Verification items for the finished model (mm, model axes). A direction names the side the tool comes from. Give positions to 0.01 mm unless a question says otherwise; leave off trailing zeros. Write each loop counter-clockwise with the first axis right and the second up, starting at its lowest first coordinate (ties: lowest second). Pieces come first, ordered by that corner, then holes. Notation, with made-up numbers: M 66.25,-14 L 77.25,-14 A17 ccw 77.25,-4 Z; hole C 89.5,40.5 d1. An arc over 180 degrees is marked long. Answer as a JSON object with one key per item and string values.
```python
from build123d import *

# Parameters (mm, degrees)
F0_W      = 76.2
F0_H      = 76.2
F1_DEPTH  = 19.05
F2_R      = 25.4
F3_DEPTH  = 76.2
F4_W      = 76.2
F4_H      = 76.2
F4_R      = 25.4
F5_DEPTH  = 19.05
F6_R      = 25.4
F7_DEPTH  = 19.05
F9_R      = 19.05
F10_DEPTH = 114.3
F8_R      = 19.05
F11_DEPTH = 608.076
F13_R     = 6.35
F14_DEPTH = 50.546


with BuildPart() as f1:
    # F0 (on Right) → F1 (new body)
    with BuildSketch(Plane.YZ):
        Rectangle(F0_W, F0_H)
    extrude(amount=F1_DEPTH)

    # F2 (on face) → F3 (join)
    with BuildSketch(Plane(origin=(0, 0, 0), x_dir=(0, -1, 0), z_dir=(-1, 0, 0))):
        Circle(F2_R)
    extrude(amount=F3_DEPTH)


with BuildPart() as f5:
    # F4 (on face) → F5 (new body)
    with BuildSketch(Plane(origin=(-76.2, 0, 0), x_dir=(0, -1, 0), z_dir=(-1, 0, 0))):
        Rectangle(F4_W, F4_H)
        Circle(F4_R, mode=Mode.SUBTRACT)
    extrude(amount=F5_DEPTH)


with BuildPart() as f7:
    # F6 (on face) → F7 (new body)
    with BuildSketch(Plane(origin=(-76.2, 0, 0), x_dir=(0, -1, 0), z_dir=(-1, 0, 0))):
        Circle(F6_R)
    extrude(amount=F7_DEPTH)


with BuildPart() as f10_tool:
    # F9 (on face) → F10 (new body)
    with BuildSketch(Plane.YZ.offset(19.05)):
        Circle(F9_R)
    extrude(amount=-F10_DEPTH)


with BuildPart() as f1_1:
    add(f1.part)

    # F10: cut by f10_tool
    add(f10_tool.part, mode=Mode.SUBTRACT)

    # F8 (on face) → F11 (cut)
    with BuildSketch(Plane(origin=(-95.25, 0, 0), x_dir=(0, -1, 0), z_dir=(-1, 0, 0))):
        Circle(F8_R)
    extrude(amount=-F11_DEPTH, mode=Mode.SUBTRACT)


with BuildPart() as f7_1:
    add(f7.part)

    # F10: cut by f10_tool
    add(f10_tool.part, mode=Mode.SUBTRACT)


with BuildPart() as f5_1:
    add(f5.part)

    # F12: union F7, F1
    add(f7_1.part)
    add(f1_1.part)

    # F13 (on face) → F14 (cut)
    with BuildSketch(Plane(origin=(-95.25, 0, 0), x_dir=(0, -1, 0), z_dir=(-1, 0, 0))):
        with Locations((-29.2046008315, -27.7056374614)):
            Circle(F13_R)
        with Locations((27.7061383014, 29.4438616986)):
            Circle(F13_R)
        with BuildLine():
            ThreePointArc((-23.0938616986, 29.4438616986), (-27.0138219031, 35.3104967301), (-33.9339897591, 33.9339897591))
            Line((-33.9339897591, 33.9339897591), (-24.9537336381, 24.9537336381))
            ThreePointArc((-24.9537336381, 24.9537336381), (-23.5772266672, 27.0138219031), (-23.0938616986, 29.4438616986))
        make_face()
        with BuildLine():
            ThreePointArc((23.3369908748, -23.3369908748), (23.455271108, -32.1957655219), (32.3140457551, -32.3140457551))
            Line((32.3140457551, -32.3140457551), (23.3369908748, -23.3369908748))
        make_face()
        with BuildLine():
            Line((23.3369908748, -23.3369908748), (32.3140457551, -32.3140457551))
            ThreePointArc((32.3140457551, -32.3140457551), (33.7790689323, -30.213783607), (34.2953991685, -27.7056374614))
            ThreePointArc((34.2953991685, -27.7056374614), (30.2968994699, -21.8070828645), (23.3369908748, -23.3369908748))
        make_face()
    extrude(amount=-F14_DEPTH, mode=Mode.SUBTRACT)


solid = f5_1.part
```
1) Section check D-D on x = 8.5. Record the boundary of the cut face in (y, z).
Completed:
{"outline": "M -38.1,-38.1 L 38.1,-38.1 L 38.1,38.1 L -38.1,38.1 Z; hole C 0,0 d38.1"}
2) Thickness scan on L1, parallel to X at y = 28.5, z = -13; L2, parallel to Z at x = -86, y = -22.5; L3, parallel to Z at x = -24.5, y = 0. Record the ranges inside material, lowest first.
Completed:
{"L1": "x = -95.25 to -76.2, 0 to 19.05", "L2": "z = -38.1 to -30.97, -24.44 to 25.81, 33.08 to 38.1", "L3": "z = -25.4 to -19.05, 19.05 to 25.4"}
3) Go/stop test with flat-tipped pins: pin 1 (6 mm diameter, centred on x = -22, y = -15.5, fed in from -Z); pin 2 (1 mm diameter, centred on x = -28, z = 18, fed in from +Y); pin 3 (7.5 mm diameter, centred on y = 29.2, z = -27.71, fed in from -X). Record where each tip stops, or that it passes through.
Completed:
{"pin 1": "stops at z = -22.11", "pin 2": "stops at y = 18.41", "pin 3": "stops at x = 0"}
4) Section check B-B on x = -85. Record the boundary of the cut face in (y, z).
Completed:
{"outline": "M -38.1,-38.1 L 38.1,-38.1 L 38.1,38.1 L -38.1,38.1 Z; hole C -27.95,-27.71 d12.7; hole C -27.71,29.44 d12.7; hole C 0,0 d38.1; hole C 29.2,-27.71 d12.7; hole M 24.95,24.95 L 33.93,33.93 A6.35 ccw Z"}
5) Section check A-A on y = 0. Record the boundary of the cut face in (x, z), and give its area (3 significant figures).
Completed:
{"outline": "M -95.25,-38.1 L -76.2,-38.1 L -76.2,-25.4 L 0,-25.4 L 0,-38.1 L 19.05,-38.1 L 19.05,-19.05 L -95.25,-19.05 Z; M -95.25,19.05 L 19.05,19.05 L 19.05,38.1 L 0,38.1 L 0,25.4 L -76.2,25.4 L -76.2,38.1 L -95.25,38.1 Z", "area": "2,420 mm2"}
6) Release check for a two-part mould opening along Y. For faces 1 (the face through (9, 38.1, -1)), 2 (the face through (-85.86, 33.88, -23.41)), 3 (the face through (-76.2, 26, 1)) record: pulls with the +Y half, pulls with the -Y half, needs draft (parallel to the pull), parting line crosses it, or undercut.
Completed:
{"face 1": "pulls with the +Y half", "face 2": "undercut", "face 3": "needs draft"}
7) Access from +Z, -Z, +X, -X, +Y, -Y to the whole of each face (thin tool, end or side, straight path). Record for faces 4 (the face through (-37.567, 5.506, -24.796)), 5 (the face through (-86, 1, -38.1)), 6 (the face through (-85.86, -33.57, 27.01)).
Completed:
{"face 4": "none", "face 5": "-Z, +X, -X, +Y, -Y", "face 6": "-X"}
